Autodesk Inventor part; units mm, degrees
ref_plane "Work Plane1" through (-2.7575, 14.1676, 33.7809) normal (0, 1, 0) x (1, 0, 0)
ref_plane "YZ Plane" through (0, 0, 0) normal (1, 0, 0) x (0, 1, 0)
ref_plane "XZ Plane" through (0, 0, 0) normal (0, 1, 0) x (-1, 0, 0)
ref_plane "Work Plane1" through (-2.7575, 14.1676, 33.7809) normal (0, 1, 0) x (1, 0, 0)
sketch "Sketch1" plane through (-2.7575, 14.1676, 33.7809) normal (0, 1, 0) x (1, 0, 0)
  line L0 (-6.2522, -27.7336) -> (82.6478, -27.7336)
  line L1 (82.6478, -27.7336) -> (82.6478, -97.5836)
  line L2 (82.6478, -97.5836) -> (-6.2522, -97.5836)
  line L3 (-6.2522, -97.5836) -> (-6.2522, -27.7336)
  point P0 (2.7575, 33.7809)
  dimension "d0" = 69.85
  dimension "d1" = 88.9
extrude "Extrusion1" add sketch "Sketch1" along normal blind 2.286
sketch "Sketch2" plane through (-2.7575, 16.4536, 33.7809) normal (0, 1, 0) x (1, 0, 0)
  line L0 (82.6478, -27.7336) -> (-6.2522, -27.7336)
  line L1 (-6.2522, -27.7336) -> (-6.2522, -97.5836)
  line L2 (-6.2522, -97.5836) -> (82.6478, -97.5836)
  line L3 (82.6478, -97.5836) -> (82.6478, -27.7336)
  circle A0 centre (5.0092, 73.556) radius 1.6383
  circle A1 centre (5.0092, 60.856) radius 1.6383
  circle A2 centre (5.0092, -2.644) radius 1.6383
  circle A3 centre (5.0092, -78.844) radius 1.6383
  circle A4 centre (5.0092, -91.544) radius 1.6383
  circle A5 centre (5.0092, -40.744) radius 1.6383
  circle A6 centre (5.0092, -53.444) radius 1.6383
  circle A7 centre (5.0092, 10.056) radius 1.6383
extrude "Extrusion2" cut sketch "Sketch2" against normal blind 2.286 contours A0 | A1 | A2 | A3 | A4 | A5 | A6 | A7
sketch "Sketch3" plane through (-2.7575, 16.4536, 33.7809) normal (0, 1, 0) x (1, 0, 0)
  line L0 (82.6478, -97.5836) -> (-6.2522, -97.5836)
  line L1 (82.6478, -27.7336) -> (-6.2522, -27.7336)
  point P0 (2.7575, 33.7809)
  point P1 (17.1634, -31.5436)
  point P2 (17.1634, -93.7736)
  dimension "d7" = 3.81
  dimension "d8" = 3.81
hole "Hole1" at (14.406, 16.4536, 65.3245) at (14.406, 16.4536, 127.5545) direction (0, -1, 0) diameter 3.2766 depth 2.286 tip angle 118
pattern_linear "Rectangular Pattern1" count 5 spacing 12.7 along (1, 0, 0) of "Hole1"
sketch "Sketch6" plane through (79.8904, 14.1676, 131.3645) normal (1, 0, 0) x (0, 0, -1)
  line L0 (69.85, 2.286) -> (0, 2.286)
  line L1 (0, 2.286) -> (0, 0)
  line L2 (0, 0) -> (69.85, 0)
  line L3 (69.85, 0) -> (69.85, 2.286)
  point P0 (131.3645, -14.1676)
extrude "Extrusion4" add sketch "Sketch6" along normal blind 2.286
fillet "Fillet2" radius 6.35 2 edges at (82.1764, 15.3106, 131.3645) (82.1764, 15.3106, 61.5145)
sketch "Sketch7" plane through (-2.7575, 16.4536, 33.7809) normal (0, 1, 0) x (1, 0, 0)
  circle A0 centre (14.7493, -82.094) radius 1.945
  circle A1 centre (76.8777, -40.2856) radius 1.905
  point P0 (2.7575, 33.7809)
extrude "Extrusion5" cut sketch "Sketch7" against normal blind 2.286
sketch "Sketch8" plane through (-2.7575, 16.4536, 33.7809) normal (0, 1, 0) x (1, 0, 0)
  circle A0 centre (18.8172, -46.9734) radius 6.35
  circle A1 centre (31.5172, -38.5914) radius 2.5732
  circle A2 centre (31.5172, -55.3554) radius 2.5732
  point P0 (2.7575, 33.7809)
  dimension "d27" = 12.7
  dimension "d33" = 12.7
  dimension "d34" = 8.382
  dimension "d35" = 8.382
extrude "Extrusion6" cut sketch "Sketch8" against normal blind 25.4
pattern_linear "Rectangular Pattern2" count 2 spacing 25.4 along (1, 0, 0) count 2 spacing 25.4 along (0, 0, 1) of "Extrusion6"
equation "\"d35\" = d34"
properties part number "talon plate short"
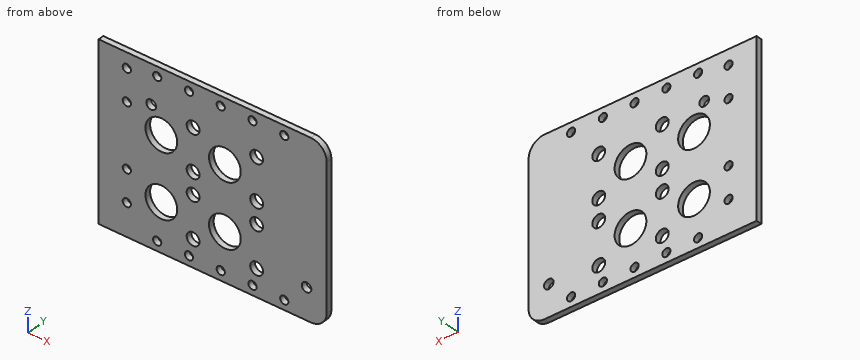
Verification items for the finished model (mm, model axes). Give positions to 0.01 mm unless a question says otherwise; leave off trailing zeros. Write each loop counter-clockwise with the first axis right and the second up, starting at its lowest first coordinate (ties: lowest second). Pieces come first, ordered by that corner, then holes.
(1) Cross-section at B-B (y = 15.25). State how many separate pieces and enclosed holes the cut face has, plus the area to 3 significant figures.
(2) Gauge pin test, flat end, axial feed: pin 1 (3 mm diameter, centred on x = 2.25, z = 112.62, fed in from +Y). Record the tip position at first contact, or that the pin passes through.
(3) Material ranges on line 1 (X direction, y = 14.85, z = 80.5); line 2 (Z direction, x = 54.5, y = 15.4); line 3 (Z direction, x = 19, y = 16.1), recorded low to high.
(4) Cross-section at A-A (z = 102). Enter the section's corners in (x, y), plus the area to 3 significant figures.
(5) Cross-section at C-C (x = 46). Enter the section's corners in (y, z).
Worked out:
1. separate pieces: 1
1. enclosed holes: 28
1. area: 5,540 mm2
2. pin 1: passes through
3. line 1: x = -9.01 to 9.71, 22.4 to 35.11, 47.8 to 82.18
3. line 2: z = 61.51 to 69.82, 74.92 to 86.59, 91.69 to 95.22, 100.32 to 111.99, 117.09 to 131.36
3. line 3: z = 61.51 to 75.13, 86.38 to 100.53, 111.78 to 131.36
4. outline: (-9.01, 14.17) - (11.26, 14.17) - (11.26, 16.45) - (-9.01, 16.45) - close; (20.86, 14.17) - (36.66, 14.17) - (36.66, 16.45) - (20.86, 16.45) - close; (46.26, 14.17) - (82.18, 14.17) - (82.18, 16.45) - (46.26, 16.45) - close
4. area: 165 mm2
5. outline: (14.17, 61.51) - (16.45, 61.51) - (16.45, 76.31) - (14.17, 76.31) - close; (14.17, 85.19) - (16.45, 85.19) - (16.45, 101.71) - (14.17, 101.71) - close; (14.17, 110.59) - (16.45, 110.59) - (16.45, 131.36) - (14.17, 131.36) - close
